from build123d import *

# Parameters (mm, degrees)
BOSS_EXTRUDE1_DEPTH = 30
BOSS_EXTRUDE2_DEPTH = 5
SKETCH3_R           = 2.5
CUT_EXTRUDE1_DEPTH  = 104.114596445


with BuildPart() as part:
    # Sketch1 → Boss-Extrude1 (new body)
    with BuildSketch(Plane(origin=(0, 0, 0), x_dir=(1, 0, 0), z_dir=(0, 1, 0))):
        with BuildLine():
            Line((0, 0), (44, 0))
            Line((44, 0), (44, 60))
            ThreePointArc((44, 60), (22, 82), (0, 60))
            Line((0, 60), (0, 0))
        make_face()
    extrude(amount=BOSS_EXTRUDE1_DEPTH)

    # Sketch2 → Boss-Extrude2 (add)
    with BuildSketch(Plane(origin=(0, 30, 0), x_dir=(1, 0, 0), z_dir=(0, 1, 0))):
        with BuildLine():
            Line((46.9, 0), (-2.9, 0))
            Line((-2.9, 0), (-2.9, 60))
            ThreePointArc((-2.9, 60), (22, 84.9), (46.9, 60))
            Line((46.9, 60), (46.9, 0))
        make_face()
    extrude(amount=BOSS_EXTRUDE2_DEPTH)

    # Sketch3 → Cut-Extrude1 (cut, through all)
    with BuildSketch(Plane(origin=(0, 35, 0), x_dir=(1, 0, 0), z_dir=(0, 1, 0))):
        with Locations(Location((22, 60, 0), (0, 0, 270))):
            Circle(SKETCH3_R)
    extrude(amount=-CUT_EXTRUDE1_DEPTH, mode=Mode.SUBTRACT)


solid = part.part
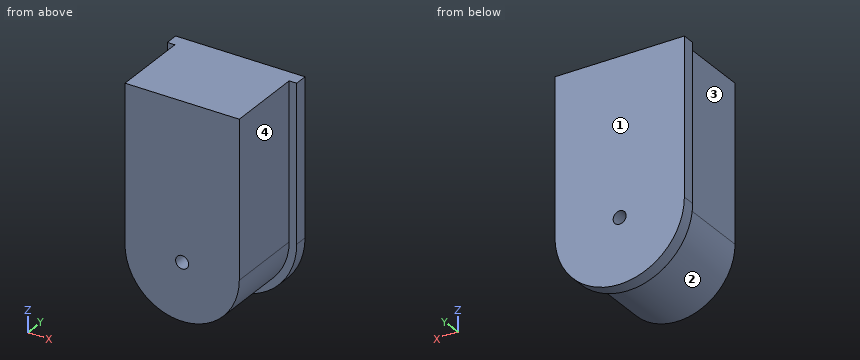
The listing builds one solid part. Answer for the finished solid, in the listing's coordinates (mm). Face numbers are marked on the shaded views. A direction names the side the tool comes from. Coordinates: 2 decimals unless noted, no trailing zeros. Order: outer loops, then holes, each group sorted by start corner. A loop starts at its lowest first (then second) coordinate and runs counter-clockwise, first axis right, second up. Notation, with made-up numbers: (45, 5) -> (77, 5) arc R19 cw to (77, 18) -> close; hole circle Ø5 at (8.25, 74.25). An arc over 180 degrees is marked (long way). Answer in a Markdown table with one row per item. Add a question column.
Item 1: Find section C-C (z = -55.5). Write down the section's boundary in (x, y).
Item 2: Find section B-B (x = 22). Write down the section's boundary in (y, z), then the cut area to 3 significant figures.
Item 3: Find section D-D (x = 34). Write down the section's boundary in (y, z), then the cut area to 3 significant figures.
Item 4: Which of the six approach directions +Z, -Z, +X, -X, +Y, -Y give full straight-line access (tool end or side, diameter ignored) to the marked faces 1, 2, 3 and 4?
Item 5: Find the intervals of material crossed by L1, parallel to X at y = 22, z = -60; L2, parallel to X at y = 17.5, z = -42.5; L3, parallel to Z at x = 22.5, y = 9.5, in increasing order. Write a range as from..to.
Item 6: Each of these flat-tipped pins is pushed along its axis until it touches: P1, Ø5, axis at x = 4, y = 8, coming from the -Z side; P2, Ø1, axis at x = 28, y = 24, coming from the -Z side; P3, Ø4, axis at y = 4.5, z = -55.5, coming from the +X side. Where does it stop, or does it pass through?
Item 7: Find section A-A (y = 21). Write down the section's boundary in (x, z), then the cut area to 3 significant figures.
Result set:
| question | item | result |
|---|---|---|
| 1 | outline | (-2.9, 30) -> (0, 30) -> (0, 0) -> (44, 0) -> (44, 30) -> (46.9, 30) -> (46.9, 35) -> (-2.9, 35) -> close |
| 2 | outline | (0, -82) -> (30, -82) -> (30, -84.9) -> (35, -84.9) -> (35, -62.5) -> (0, -62.5) -> close; (0, -57.5) -> (35, -57.5) -> (35, 0) -> (0, 0) -> close |
| 2 | area | 2,710 mm² |
| 3 | outline | (0, -78.44) -> (30, -78.44) -> (30, -81.82) -> (35, -81.82) -> (35, 0) -> (0, 0) -> close |
| 3 | area | 2,760 mm² |
| 4 | face 1 | +Z, -Z, +X, -X, +Y |
| 4 | face 2 | -Z, -Y |
| 4 | face 3 | +Z, -Z, -X, -Y |
| 4 | face 4 | +Z, -Z, +X, -Y |
| 5 | L1 | x = 0..19.5, 24.5..44 |
| 5 | L2 | x = 0..44 |
| 5 | L3 | z = -81.99..-62.45, -57.55..0 |
| 6 | P1 | stops at z = -75.61 |
| 6 | P2 | stops at z = -81.3 |
| 6 | P3 | stops at x = 44 |
| 7 | outline | (0, -60) arc R22 ccw to (44, -60) -> (44, 0) -> (0, 0) -> close; hole circle Ø5 at (22, -60) |
| 7 | area | 3,380 mm² |
